Could you check a few things on this model? Use its own coordinates, in mm. Coordinates: 2 decimals unless noted, no trailing zeros. Loops run counter-clockwise (first coordinate to the right, second up) from the corner with the lowest first, then second, coordinate; pieces in that order, holes last.
from build123d import *

# Parameters (mm, degrees)
F2_DEPTH = 31
F3_DEPTH = 12
F4_R     = 2


with BuildPart() as f2:
    # F1 (on Top) → F2 (new body)
    with BuildSketch(Plane.XY):
        Polygon((-19, 0.5), (-21, 0.5), (-21, -0.5), (-19, -0.5), (19, -0.5), (21, -0.5), (21, 0.5), (19, 0.5), align=None)
    extrude(amount=F2_DEPTH)

    # F1 (on Top) → F3 (join)
    with BuildSketch(Plane.XY):
        Polygon((-21, 0.75), (-21, 0.5), (-19, 0.5), align=None)
        Polygon((-19, -0.5), (-21, -0.5), (-21, -0.75), align=None)
        Polygon((21, 0.75), (19, 0.5), (21, 0.5), align=None)
        Polygon((21, -0.5), (19, -0.5), (21, -0.75), align=None)
    extrude(amount=F3_DEPTH)

    # F4
    f4_edges = [f2.edges().sort_by_distance(p)[0] for p in [
        (-21, 0, 31),
        (21, 0, 31),
    ]]
    fillet(f4_edges, radius=F4_R)


solid = f2.part
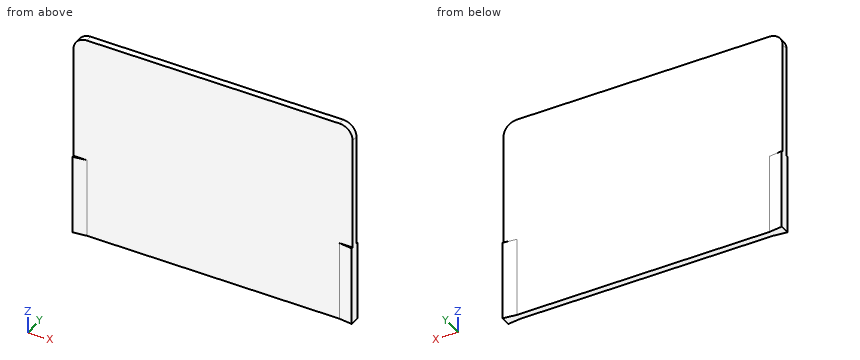
(1) Imagine slicing it at C-C, the plane z = 15. Write out the boundary of the cut face in (x, y).
Answers:
outline: (-21, -0.5) - (21, -0.5) - (21, 0.5) - (-21, 0.5) - close
(2) For pin 1 (4 mm diameter, centred on x = 9, z = 28, fed in from -Y), with a flat end and sliding along its axis, tell me the tip position at first contact or that it passes through.
Answers:
pin 1: stops at y = -0.5
(3) I need wall thicknesses on probe 1 along Y at (x, z) = (-9, 8.5). Which ranges of the line are inside material? Lowest first, please.
Answers:
probe 1: y = -0.5 to 0.5
(4) Imagine slicing it at B-B, the plane x = -9. Write out the boundary of the cut face in (y, z), and give its area (3 significant figures).
Answers:
outline: (-0.5, 0) - (0.5, 0) - (0.5, 31) - (-0.5, 31) - close
area: 31.0 mm2
(5) Imagine slicing it at A-A, the plane z = 6. Write out the boundary of the cut face in (x, y).
Answers:
outline: (-21, -0.75) - (-19, -0.5) - (19, -0.5) - (21, -0.75) - (21, 0.75) - (19, 0.5) - (-19, 0.5) - (-21, 0.75) - close
